Geometry check sheet. Reference: drawing and pictorial views, mm from the part's lowest x, y, z. A direction names the side the tool comes from. Round coordinates to 2 decimals unless told otherwise and drop trailing zeros. Write each loop counter-clockwise with the first axis right and the second up, starting at its lowest first coordinate (ties: lowest second). Pieces come first, ordered by that corner, then holes. Notation, with made-up numbers: M 57.5,56 L 92.5,56 A29 ccw 92.5,94 Z; hole C -39.75,48 d11. An arc over 180 degrees is marked long. Put each result on its own line as item: value. Start each with the question number.
(1) Section check C-C on y = 5.25. Record the cut outline in (x, z).
(2) Section check B-B on z = 12.5. Record the cut outline in (x, y).
(3) Section check A-A on x = 12.5. Record the cut outline in (y, z).
(4) Material ranges on probe 1 along Y at (x, z) = (2.75, 12.5); probe 2 along X at (y, z) = (2.25, 13) (1 decimal); probe 3 along X at (y, z) = (7.5, 12.5), recorded low to high.
(5) Mould release check, pull along X, two halves, no side actions. Record for the marked faces 3, 4 and 5: pulls with the +X half, pulls with the -X half, needs draft (parallel to the pull), parting line crosses it, or undercut.
(6) Tool access check on the marked faces 1 and 2. Record the directions out of +Z, -Z, +X, -X, +Y, -Y that give a thin tool (end or side, any length) a straight path to the whole face; none if there is none.
(7) Section check D-D on y = 1.5. Record the cut outline in (x, z).
(8) Gauge pin test, flat ends, axial feed: pin 1 (2 mm diameter, centred on x = 19.76, z = 12.5, fed in from +Y); pin 2 (2 mm diameter, centred on x = 8.5, z = 21, fed in from +Y); pin 3 (7 mm diameter, centred on x = 9.5, z = 10, fed in from +Y); pin 4 (1.5 mm diameter, centred on x = 20.5, y = 3.5, fed in from -Z). Record the tip position at first contact, or that the pin passes through.
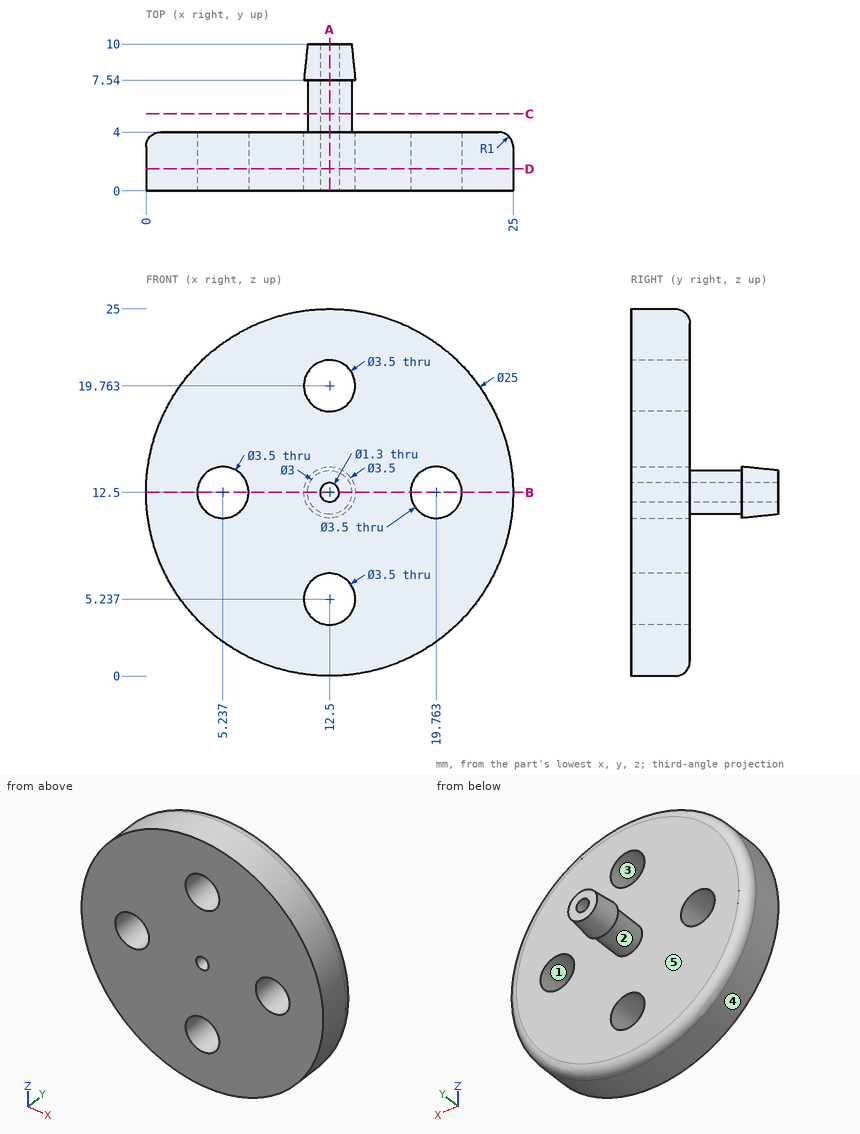
Answers follow:
1. outline: C 12.5,12.5 d3; hole C 12.5,12.5 d1.3
2. outline: M 0,0 L 3.49,0 L 3.49,4 L 1,4 A1 ccw 0,3 Z; M 6.99,0 L 11.85,0 L 11.85,10 L 11,10 L 10.75,7.54 L 11,7.54 L 11,4 L 6.99,4 Z; M 13.15,0 L 18.01,0 L 18.01,4 L 14,4 L 14,7.54 L 14.25,7.54 L 14,10 L 13.15,10 Z; M 21.51,0 L 25,0 L 25,3 A1 ccw 24,4 L 21.51,4 Z
3. outline: M 0,0 L 3,0 A1 ccw 4,1 L 4,3.49 L 0,3.49 Z; M 0,6.99 L 4,6.99 L 4,11 L 7.54,11 L 7.54,10.75 L 10,11 L 10,11.85 L 0,11.85 Z; M 0,13.15 L 10,13.15 L 10,14 L 7.54,14.25 L 7.54,14 L 4,14 L 4,18.01 L 0,18.01 Z; M 0,21.51 L 4,21.51 L 4,24 A1 ccw 3,25 L 0,25 Z
4. probe 1: y = 0 to 4
4. probe 2: x = 0 to 3.6, 6.9 to 12.1, 12.9 to 18.1, 21.4 to 25
4. probe 3: x = 11 to 11.85, 13.15 to 14
5. face 3: undercut
5. face 4: parting line crosses it
5. face 5: needs draft
6. face 1: +Y, -Y
6. face 2: none
7. outline: C 12.5,12.5 d25; hole C 5.24,12.5 d3.5; hole C 12.5,5.24 d3.5; hole C 12.5,19.76 d3.5; hole C 12.5,12.5 d1.3; hole C 19.76,12.5 d3.5
8. pin 1: passes through
8. pin 2: stops at y = 4
8. pin 3: stops at y = 10
8. pin 4: stops at z = 2.39
